Build history of the part. All positions in model axes, mm. Round coordinates to 2 decimals unless told otherwise and drop trailing zeros. Write each loop counter-clockwise with the first axis right and the second up, starting at its lowest first coordinate (ties: lowest second). Pieces come first, ordered by that corner, then holes.
from build123d import *

# Parameters (mm, degrees)
SKETCH1_W           = 100
SKETCH1_H           = 10
BOSS_EXTRUDE1_DEPTH = 1.5
SKETCH2_R           = 1
CUT_EXTRUDE2_DEPTH  = 2
SKETCH5_W           = 6
SKETCH5_H           = 2
SKETCH5_W_2         = 3
SKETCH5_H_2         = 6
CUT_EXTRUDE4_DEPTH  = 2


with BuildPart() as part:
    # Sketch1 → Boss-Extrude1 (new body)
    with BuildSketch(Plane(origin=(0, 0, 0), x_dir=(1, 0, 0), z_dir=(0, 1, 0))):
        with Locations((40.170187286, 0.880693734)):
            Rectangle(SKETCH1_W, SKETCH1_H)
    extrude(amount=BOSS_EXTRUDE1_DEPTH)

    # Sketch2 → Cut-Extrude2 (cut)
    with BuildSketch(Plane(origin=(0, 1.5, 0), x_dir=(1, 0, 0), z_dir=(0, 1, 0))):
        with Locations((40.170187286, 0.880693734)):
            Circle(SKETCH2_R)
    extrude(amount=-CUT_EXTRUDE2_DEPTH, mode=Mode.SUBTRACT)

    # Sketch5 → Cut-Extrude4 (cut)
    with BuildSketch(Plane(origin=(0, 1.5, 0), x_dir=(1, 0, 0), z_dir=(0, 1, 0))):
        with Locations((40.170187286, 4.880693734)):
            Rectangle(SKETCH5_W, SKETCH5_H)
        with Locations((40.170187286, -3.119306266)):
            Rectangle(SKETCH5_W, SKETCH5_H)
        with Locations((-6.329812714, 0.880693734)):
            Rectangle(SKETCH5_W_2, SKETCH5_H_2)
        with Locations((86.670187286, 0.880693734)):
            Rectangle(SKETCH5_W_2, SKETCH5_H_2)
    extrude(amount=-CUT_EXTRUDE4_DEPTH, mode=Mode.SUBTRACT)


solid = part.part
1) Wall check: L1, parallel to X at y = 0.55, z = 2; L2, parallel to X at y = 0.4, z = -1; L3, parallel to X at y = 0.1, z = 3.5. Give the ranges that are in metal, low to high.
Results:
L1: x = -9.83 to -7.83, -4.83 to 85.17, 88.17 to 90.17
L2: x = -9.83 to -7.83, -4.83 to 39.18, 41.16 to 85.17, 88.17 to 90.17
L3: x = -9.83 to 37.17, 43.17 to 90.17
2) Slice it at B-B (y = 0.9). Write the cut outline in (x, z).
Results:
outline: (-9.83, -5.88) - (37.17, -5.88) - (37.17, -3.88) - (43.17, -3.88) - (43.17, -5.88) - (90.17, -5.88) - (90.17, 4.12) - (43.17, 4.12) - (43.17, 2.12) - (37.17, 2.12) - (37.17, 4.12) - (-9.83, 4.12) - close; hole (-7.83, -3.88) - (-4.83, -3.88) - (-4.83, 2.12) - (-7.83, 2.12) - close; hole circle Ø2 at (40.17, -0.88); hole (85.17, -3.88) - (88.17, -3.88) - (88.17, 2.12) - (85.17, 2.12) - close
3) Pin check, flat tip, straight feed: pin 1 Ø0.8 at (x, y) = (40.5, 1) entering from -Z. Stop position of the tip, or through.
Results:
pin 1: stops at z = -3.88
4) Slice it at A-A (z = 1). Write the cut outline in (x, y), plus the area to 3 significant figures.
Results:
outline: (-9.83, 0) - (-7.83, 0) - (-7.83, 1.5) - (-9.83, 1.5) - close; (-4.83, 0) - (85.17, 0) - (85.17, 1.5) - (-4.83, 1.5) - close; (88.17, 0) - (90.17, 0) - (90.17, 1.5) - (88.17, 1.5) - close
area: 141 mm2
5) Slice it at C-C (x = 42). Write the cut outline in (y, z).
Results:
outline: (0, -3.88) - (1.5, -3.88) - (1.5, 2.12) - (0, 2.12) - close
6) Mould opens along Z. For faces 1 (the cylindrical face through (39.17, 0.76, -0.92)), 2 (the flat face through (39, 1.5, -2)) say: released by +Z, released by -Z, zero draft, split by the parting line, or undercut.
Results:
face 1: undercut
face 2: zero draft
